Answer from the drawing. Dimensions are ordinates in mm from the lowest x, y and z of the part. Give positions to 0.01 mm unless a question says otherwise; leave off trailing zeros. Write each loop counter-clockwise with the first axis right and the second up, starting at its lowest first coordinate (ties: lowest second). Pieces come first, ordered by that corner, then holes. Notation, with made-up numbers: (51.25, 69.5) -> (70.25, 69.5) arc R8 ccw to (70.25, 77.5) -> close; hole circle Ø2 at (1.25, 79.25). An arc over 180 degrees is marked (long way). Write item = value, one per line.
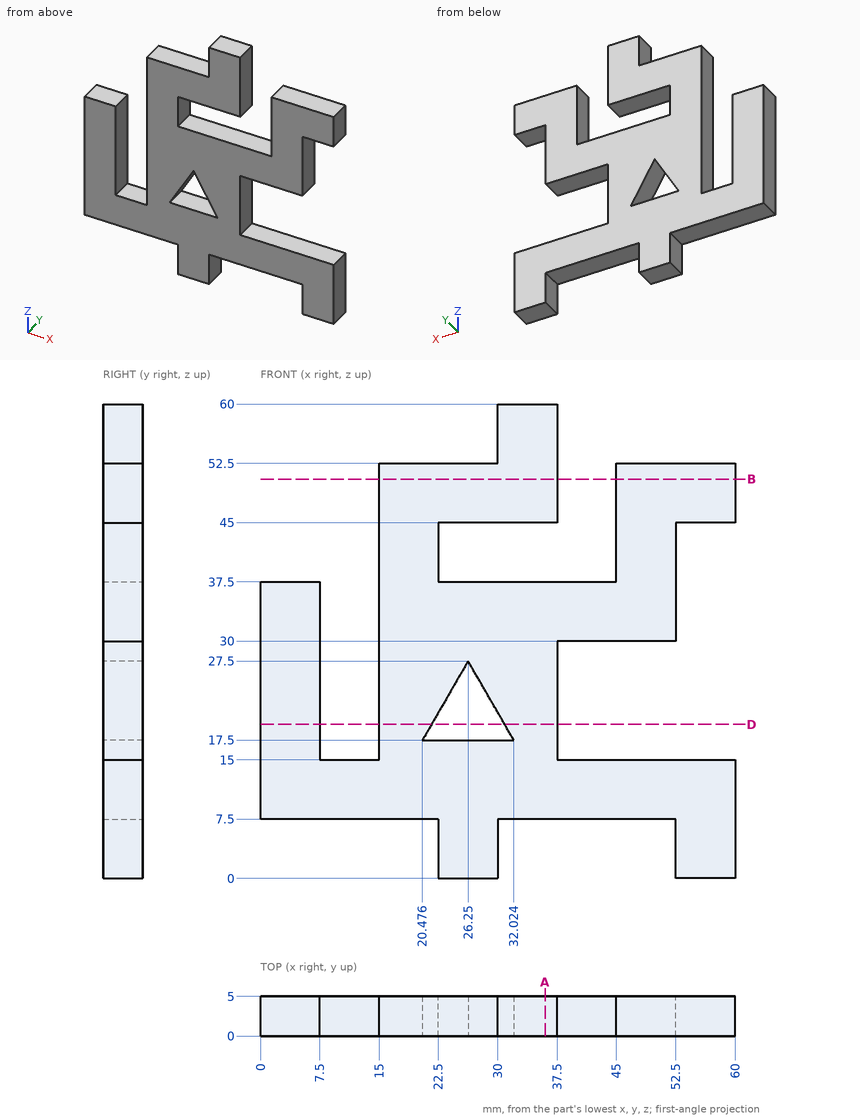
(1) Consider L1, parallel to X at y = 2.75, z = 40; L2, parallel to X at y = 2.5, z = 15.5; L3, parallel to Z at x = 25.5, y = 2 (1 decimal). Determine where each line is inside the solid, lowest interval first.
Checks:
L1 = 15 to 22.5, 45 to 52.5
L2 = 0 to 7.5, 15 to 37.5
L3 = 0 to 17.5, 26.2 to 37.5, 45 to 52.5
(2) The part is cut by section D-D on z = 19.5. Determine the outline of the cut face in (x, y).
Checks:
outline = (0, 0) -> (7.5, 0) -> (7.5, 5) -> (0, 5) -> close; (15, 0) -> (21.63, 0) -> (21.63, 5) -> (15, 5) -> close; (30.87, 0) -> (37.5, 0) -> (37.5, 5) -> (30.87, 5) -> close
(3) The part is cut by section A-A on x = 36. Determine the outline of the cut face in (y, z).
Checks:
outline = (0, 7.5) -> (5, 7.5) -> (5, 37.5) -> (0, 37.5) -> close; (0, 45) -> (5, 45) -> (5, 60) -> (0, 60) -> close
(4) The part is cut by section B-B on z = 50.5. Determine the outline of the cut face in (x, y).
Checks:
outline = (15, 0) -> (37.5, 0) -> (37.5, 5) -> (15, 5) -> close; (45, 0) -> (60, 0) -> (60, 5) -> (45, 5) -> close
(5) Given P1, Ø1, axis at x = 26.5, z = 9.5, coming from the -Y side; P2, Ø2.5, axis at x = 20.5, y = 2, coming from the +Z side; P3, Ø3, axis at y = 3, z = 40, coming from the -X side; P4, Ø1.5, axis at x = 31, y = 2.5, coming from the -Z side, each flat-ended and moving along its own axis, determine where each tip first touches the part or whether it passes through.
Checks:
P1 = 0
P2 = 52.5
P3 = 15
P4 = 7.5
